Model file for the job. Use its own axes, mm. Face numbers are marked on the shaded views. A direction names the side the tool comes from. Coordinates: 2 decimals unless noted, no trailing zeros. Write each loop counter-clockwise with the first axis right and the second up, starting at its lowest first coordinate (ties: lowest second). Pieces come first, ordered by that corner, then holes. Notation, with made-up numbers: M -29.5,89 L -0.5,89 A27 cw -0.5,108 Z; hole C 56,72 d2. An arc over 180 degrees is marked long. One line per question, with ' | ' between items. Start each with the question number.
(1) Tool access for the marked faces 4, 5 and 6: list every direction of +Z, -Z, +X, -X, +Y, -Y with a clear straight run to the whole face (end or side of a thin tool).
(2) Flat gauge pins, fed straight in: pin 1 Ø3 at (x, z) = (-3.5, -5) entering from +Y; pin 2 Ø1.2 at (x, z) = (0, 4) entering from -Y. Where does each tip first touch, or does it go through?
(3) Wall check: probe 1 along X at (y, z) = (1.6, -0.75); probe 2 along X at (y, z) = (0.6, 3.75); probe 3 along Y at (x, z) = (-7.25, -1.8). Give the ranges that are in metal, low to high.
(4) Cut at A-A (z = -2.25). Write the cut outline in (x, y), plus the area to 3 significant figures.
(5) Cut at C-C (y = 2.5). Write the cut outline in (x, z).
(6) Cut at D-D (x = 6). Write the cut outline in (y, z).
(7) Cut at B-B (z = -8.75). Write the cut outline in (x, y), plus the area to 3 significant figures.
(8) Two-plate mould, pull along X, no slides. Class the marked faces 1, 2 and 3: +X half, -X half, draft (parallel to the pull), parting line (faces both ways), or undercut.
from build123d import *

# Parameters (mm, degrees)
SKETCH1_W           = 25
SKETCH1_H           = 9.6
BOSS_EXTRUDE1_DEPTH = 5
SKETCH2_W           = 10.6
SKETCH2_H           = 7.3
CUT_EXTRUDE1_DEPTH  = 10
SKETCH3_W           = 7.3
SKETCH3_H           = 1.98
CUT_EXTRUDE2_DEPTH  = 10
SKETCH4_R           = 0.75
CUT_EXTRUDE3_DEPTH  = 26
SKETCH6_W           = 7.2
SKETCH6_H           = 5
BOSS_EXTRUDE3_DEPTH = 5.5


with BuildPart() as part:
    # Sketch1 → Boss-Extrude1 (new body)
    with BuildSketch(Plane(origin=(0, 0, 0), x_dir=(1, 0, 0), z_dir=(0, 1, 0))):
        Rectangle(SKETCH1_W, SKETCH1_H)
    extrude(amount=BOSS_EXTRUDE1_DEPTH)

    # Sketch2 → Cut-Extrude1 (cut)
    with BuildSketch(Plane(origin=(0, 5, 0), x_dir=(1, 0, 0), z_dir=(0, 1, 0))):
        with Locations((0, 1.15)):
            Rectangle(SKETCH2_W, SKETCH2_H)
    extrude(amount=-CUT_EXTRUDE1_DEPTH, mode=Mode.SUBTRACT)

    # Sketch3 → Cut-Extrude2 (cut)
    with BuildSketch(Plane(origin=(0, 0, 2.5), x_dir=(-1, 0, 0), z_dir=(0, 0, -1))):
        with Locations((-0.2, 0.99)):
            Rectangle(SKETCH3_W, SKETCH3_H)
    extrude(amount=-CUT_EXTRUDE2_DEPTH, mode=Mode.SUBTRACT)

    # Sketch4 → Cut-Extrude3 (cut)
    with BuildSketch(Plane.ZY.offset(12.5)):
        with Locations((-1.8, 2.5)):
            Circle(SKETCH4_R)
    extrude(amount=-CUT_EXTRUDE3_DEPTH, mode=Mode.SUBTRACT)

    # Sketch6 → Boss-Extrude3 (add)
    with BuildSketch(Plane(origin=(0, 0, -4.8), x_dir=(-1, 0, 0), z_dir=(0, 0, -1))):
        with Locations((-8.9, 2.5)):
            Rectangle(SKETCH6_W, SKETCH6_H)
        with Locations((8.9, 2.5)):
            Rectangle(SKETCH6_W, SKETCH6_H)
    extrude(amount=BOSS_EXTRUDE3_DEPTH)


solid = part.part
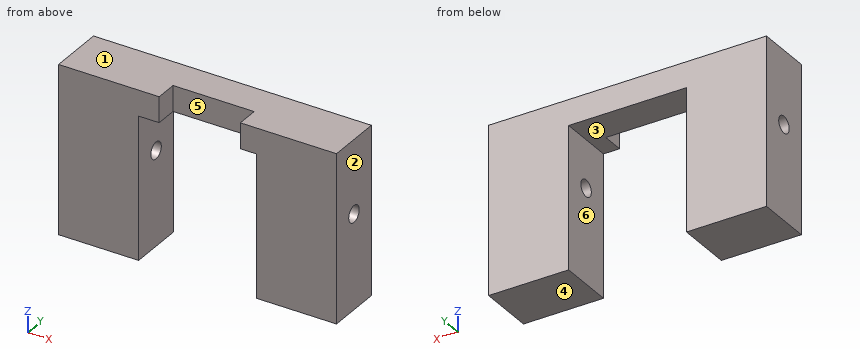
Filled in:
1) face 4: -Z, +X, -X, +Y, -Y | face 5: +Z, -Z, -Y | face 6: -Z, +Y, -Y
2) pin 1: through | pin 2: y = 1.98
3) probe 1: -12.5 to -5.3, 5.3 to 12.5 | probe 2: -12.5 to -3.45, 3.85 to 12.5 | probe 3: 0 to 1.75, 3.25 to 5
4) outline: M -12.5,0 L -5.3,0 L -5.3,1.9 L -12.5,1.9 Z; M -12.5,3.1 L -5.3,3.1 L -5.3,5 L -12.5,5 Z; M 5.3,0 L 12.5,0 L 12.5,1.9 L 5.3,1.9 Z; M 5.3,3.1 L 12.5,3.1 L 12.5,5 L 5.3,5 Z | area: 54.7 mm²
5) outline: M -12.5,-10.3 L -5.3,-10.3 L -5.3,-2.55 L -12.5,-2.55 Z; M -12.5,-1.05 L -5.3,-1.05 L -5.3,2.5 L 5.3,2.5 L 5.3,-1.05 L 12.5,-1.05 L 12.5,4.8 L -12.5,4.8 Z; M 5.3,-10.3 L 12.5,-10.3 L 12.5,-2.55 L 5.3,-2.55 Z
6) outline: M 0,-10.3 L 5,-10.3 L 5,4.8 L 0,4.8 Z; hole C 2.5,-1.8 d1.5
7) outline: M -12.5,0 L -5.3,0 L -5.3,5 L -12.5,5 Z; M 5.3,0 L 12.5,0 L 12.5,5 L 5.3,5 Z | area: 72.0 mm²
8) face 1: draft | face 2: +X half | face 3: undercut
